from build123d import *

# Parameters (mm, degrees)
ESQUISSE1_W            = 39
ESQUISSE1_H            = 33
BOSS_EXTRU_1_DEPTH     = 1
ESQUISSE2_W            = 29.92
ESQUISSE2_H            = 35.92
ESQUISSE2_W_2          = 27.92
ESQUISSE2_H_2          = 33.92
BOSS_EXTRU_2_DEPTH     = 1
R_VOLUTION2_ANGLE      = 180
SYM_TRIE2_COPY_1_ANGLE = 180
CONG_1_R               = 1
CONG_2_R               = 1


with BuildPart() as part:
    # Esquisse1 → Boss.-Extru.1 (new body)
    with BuildSketch(Plane(origin=(0, 0, 0), x_dir=(0, 1, 0), z_dir=(0, 0, 1))):
        Rectangle(ESQUISSE1_W, ESQUISSE1_H)
    extrude(amount=BOSS_EXTRU_1_DEPTH)

    # Esquisse2 → Boss.-Extru.2 (add)
    with BuildSketch(Plane.XY.offset(1)):
        Rectangle(ESQUISSE2_W, ESQUISSE2_H)
        Rectangle(ESQUISSE2_W_2, ESQUISSE2_H_2, mode=Mode.SUBTRACT)
    extrude(amount=BOSS_EXTRU_2_DEPTH)

    # Esquisse3 → Révolution2 (revolve)
    with BuildSketch(Plane.YZ.offset(14.96)):
        with BuildLine():
            Line((-9.31, 1.5), (-8.61, 1.5))
            ThreePointArc((-8.61, 1.5), (-8.96, 1.85), (-9.31, 1.5))
        make_face()
    r_volution2 = revolve(axis=Axis((14.96, -17.96, 1.5), (0, 1, 0)), revolution_arc=R_VOLUTION2_ANGLE)

    # Symétrie1: Révolution2 across plane
    add(r_volution2.mirror(Plane.ZX))

    # Symétrie2: Révolution2 across plane
    add(r_volution2.mirror(Plane(origin=(0, 0, 0), x_dir=(0, 0, 1), z_dir=(1, 0, 0))))

    # Symétrie2 copy 1 sketch → Symétrie2 copy 1 (revolve)
    with BuildSketch(Plane(origin=(-14.96, 0, 0), x_dir=(0, -1, 0), z_dir=(-1, 0, 0))):
        with BuildLine():
            Line((-9.31, 1.5), (-8.61, 1.5))
            ThreePointArc((-8.61, 1.5), (-8.96, 1.85), (-9.31, 1.5))
        make_face()
    revolve(axis=Axis((-14.96, 17.96, 1.5), (0, -1, 0)), revolution_arc=SYM_TRIE2_COPY_1_ANGLE)

    # Congé1
    cong_1_edges = [part.edges().sort_by_distance(p)[0] for p in [
        (16.5, 19.5, 0.5),
        (16.5, -19.5, 0.5),
        (-16.5, -19.5, 0.5),
        (-16.5, 19.5, 0.5),
    ]]
    fillet(cong_1_edges, radius=CONG_1_R)

    # Congé2
    cong_2_edges = [part.edges().sort_by_distance(p)[0] for p in [
        (14.96, 17.96, 1.5),
        (-14.96, 17.96, 1.5),
        (-14.96, -17.96, 1.5),
        (14.96, -17.96, 1.5),
    ]]
    fillet(cong_2_edges, radius=CONG_2_R)


solid = part.part
CAD build for the part. Positions are in the model's coordinates, mm. A direction names the side the tool comes from. Round coordinates to 2 decimals unless told otherwise and drop trailing zeros. Order: outer loops, then holes, each group sorted by start corner. A loop starts at its lowest first (then second) coordinate and runs counter-clockwise, first axis right, second up. Notation, with made-up numbers: M 30,-14 L 86,-14 A16 ccw 86,9 Z; hole C 65.25,13.5 d11. An arc over 180 degrees is marked long. Use one line per item in the form item = value.
Q1. Saw through at B-B on y = 0. Give the cut face in (x, z), then the cut area to 3 significant figures.
Recorded:
outline = M -16.5,0 L 16.5,0 L 16.5,1 L 14.96,1 L 14.96,2 L 13.96,2 L 13.96,1 L -13.96,1 L -13.96,2 L -14.96,2 L -14.96,1 L -16.5,1 Z
area = 35.0 mm^2
Q2. Flat gauge pins, fed straight in: P1, Ø0.5, axis at y = -4, z = 1.5, coming from the -X side; P2, Ø0.5, axis at y = -5.5, z = 1.5, coming from the +X side; P3, Ø3, axis at x = 12, y = -8.5, coming from the +Z side; P4, Ø12, axis at x = 5, y = -2, coming from the -Z side. Where does each tip first touch, or does it go through?
Recorded:
P1 = -14.96
P2 = 14.96
P3 = 1
P4 = 0
Q3. Two-plate mould, pull along Y, no slides. Class faces 4 (the flat face through (-0.2, 16.96, 1.5)), 5 (the flat face through (13.96, -0.2, 1.5)), 6 (the cylindrical face through (-14.659, 17.675, 1.507)), 7 (the cylindrical face through (16.199, -19.215, 0.507)): +Y half, -Y half, draft (parallel to the pull), parting line (faces both ways), or undercut.
Recorded:
face_4 = undercut
face_5 = undercut
face_6 = +Y half
face_7 = -Y half
Q4. Which spindle directions (+Z, -Z, +X, -X, +Y, -Y) get a long thin tool onto all of the face, cutting with end or side? Do faces 1 (the cylindrical face through (14.675, 17.659, 1.507)), 2 (the cylindrical face through (-14.659, -17.675, 1.507)), 3 (the cylindrical face through (14.659, -17.675, 1.507)). Say none if no direction does.
Recorded:
face_1 = +Z, +X, +Y
face_2 = +Z, -X, -Y
face_3 = +Z, +X, -Y
Q5. Saw through at A-A on x = -11. Give the cut face in (y, z).
Recorded:
outline = M -19.5,0 L 19.5,0 L 19.5,1 L 17.96,1 L 17.96,2 L 16.96,2 L 16.96,1 L -16.96,1 L -16.96,2 L -17.96,2 L -17.96,1 L -19.5,1 Z
Q6. Probe L1, parallel to Y at x = 9.5, z = 1.15; L2, parallel to X at y = -15, z = 1.8; L3, parallel to Z at x = -12.5, y = 3. List the from-to ranges inside material, lowest first.
Recorded:
L1 = -17.96 to -16.96, 16.96 to 17.96
L2 = -14.96 to -13.96, 13.96 to 14.96
L3 = 0 to 1
